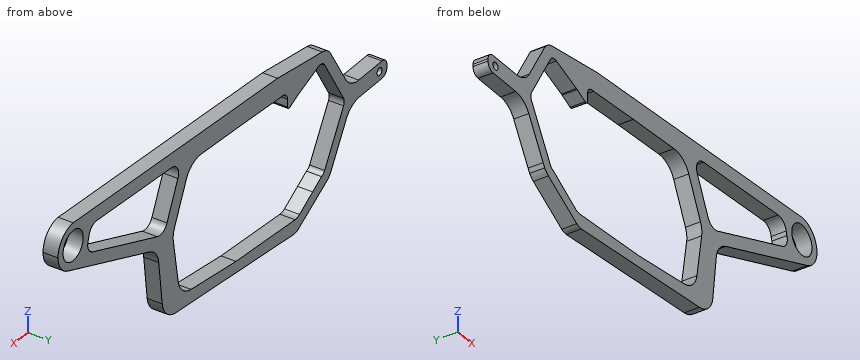
from build123d import *

# Parameters (mm, degrees)
F1_R     = 1
F1_R_2   = 4
F2_DEPTH = 4


# Not quite as in the source:
# - a feature names something its author has since deleted; it is built from what else it names


with BuildPart() as f2:
    # F1 (on Front) → F2 (new body)
    with BuildSketch(Plane.XZ):
        with BuildLine():
            ThreePointArc((53.6725900561, -3.4803708923), (56.4360817028, -1.2749098512), (57.4778270766, 2.1038045583))
            ThreePointArc((57.4778270766, 2.1038045583), (55.7204672392, 6.3464457699), (51.4778255932, 8.1038045583))
            Line((51.4778255932, 8.1038045583), (-29.5767494715, 1.8164854333))
            Line((-29.5767494715, 1.8164854333), (-47.2952228074, -0.9563085456))
            ThreePointArc((-47.2952228074, -0.9563085456), (-48.9181443858, -1.5076422035), (-50.2595064205, -2.5746900675))
            Line((-50.2595064205, -2.5746900675), (-56.5978536574, -13.3921147633))
            ThreePointArc((-56.5978536574, -13.3921147633), (-58.7913353541, -15.5645829823), (-61.7746472195, -16.3588313254))
            Line((-61.7746472195, -16.3588313254), (-70.9623719458, -16.3588313254))
            ThreePointArc((-70.9623719458, -16.3588313254), (-72.3660357626, -16.9341461359), (-72.9621509967, -18.3291034361))
            Line((-72.9621509967, -18.3291034361), (-72.9714351561, -18.9536438246))
            ThreePointArc((-72.9714351561, -18.9536438246), (-72.3963412947, -20.3870355307), (-70.9716561052, -20.9833717139))
            Line((-70.9716561052, -20.9833717139), (-62.0211355409, -20.9833717139))
            ThreePointArc((-62.0211355409, -20.9833717139), (-59.0238889239, -21.7856305971), (-56.8281648814, -23.977867475))
            Line((-56.8281648814, -23.977867475), (-51.1217613336, -33.8375062708))
            Line((-51.1217613336, -33.8375062708), (-50.5134866975, -34.8884954183))
            ThreePointArc((-50.5134866975, -34.8884954183), (-49.834113752, -35.622752626), (-49.0221729234, -36.2070755993))
            Line((-49.0221729234, -36.2070755993), (-37.7895467449, -42.6922353472))
            ThreePointArc((-37.7895467449, -42.6922353472), (-36.9110233024, -43.029081092), (-35.9713694581, -43.0772386209))
            Line((-35.9713694581, -43.0772386209), (10.8377953956, -38.0845412605))
            ThreePointArc((10.8377953956, -38.0845412605), (14.4191592098, -36.3857997297), (16.1597362046, -32.824580657))
            Line((16.1597362046, -32.824580657), (17.5522645357, -21.0756224064))
            ThreePointArc((17.5522645357, -21.0756224064), (18.760112016, -18.1166816586), (21.3157969388, -16.1976453223))
            Line((21.3157969388, -16.1976453223), (53.6725900561, -3.4803708923))
        make_face()
        with Locations((-70.0084173118, -18.6587822488)):
            Circle(F1_R, mode=Mode.SUBTRACT)
        with BuildLine():
            ThreePointArc((-33.5221489054, -5.8863848639), (-32.7820426942, -4.3428905644), (-31.1190403454, -3.9372367165))
            Line((-31.1190403454, -3.9372367165), (-15.3857114758, -2.6969403245))
            ThreePointArc((-15.3857114758, -2.6969403245), (-15.3533597704, -2.6945658839), (-15.320984282, -2.6925413929))
            Line((-15.320984282, -2.6925413929), (0.7603415418, -1.5996367209))
            ThreePointArc((0.7603415418, -1.5996367209), (4.2304854801, -2.4267493449), (6.6177460931, -5.0775984562))
            Line((6.6177460931, -5.0775984562), (11.2725159026, -15.1927708333))
            ThreePointArc((11.2725159026, -15.1927708333), (11.7672314644, -16.8926047847), (11.7443467828, -18.6628181167))
            Line((11.7443467828, -18.6628181167), (9.8637327358, -30.2427322728))
            ThreePointArc((9.8637327358, -30.2427322728), (8.1254532697, -33.5812724587), (4.7405491326, -35.2274468291))
            Line((4.7405491326, -35.2274468291), (-13.1016644536, -37.6254695609))
            Line((-13.1016644536, -37.6254695609), (-36.5010263621, -39.4700978904))
            ThreePointArc((-36.5010263621, -39.4700978904), (-37.4240833549, -39.3995872417), (-38.2816944982, -39.0510057009))
            Line((-38.2816944982, -39.0510057009), (-43.475593846, -35.9307785793))
            Line((-43.475593846, -35.9307785793), (-46.9845830439, -33.8227586638))
            ThreePointArc((-46.9845830439, -33.8227586638), (-47.7169758073, -33.480833261), (-48.2542237632, -32.8769485246))
            Line((-48.2542237632, -32.8769485246), (-55.7535278454, -19.8877718654))
            ThreePointArc((-55.7535278454, -19.8877718654), (-56.0221729234, -18.8865675237), (-55.7535278454, -17.8853631819))
            Line((-55.7535278454, -17.8853631819), (-48.3466238348, -5.0768093424))
            ThreePointArc((-48.3466238348, -5.0768093424), (-47.2942991525, -4.0512417288), (-45.8251853322, -4.0215642922))
            Line((-45.8251853322, -4.0215642922), (-37.9265817129, -6.9582780391))
            Line((-37.9265817129, -6.9582780391), (-37.6259790546, -7.0700425992))
            Line((-37.6259790546, -7.0700425992), (-34.4656276648, -8.5558833842))
            ThreePointArc((-34.4656276648, -8.5558833842), (-33.8292769309, -8.5156852397), (-33.5221489054, -7.9569093245))
            Line((-33.5221489054, -7.9569093245), (-33.5221489054, -5.9059880699))
            ThreePointArc((-33.5221489054, -5.9059880699), (-33.5221729234, -5.8961864669), (-33.5221489054, -5.8863848639))
        make_face(mode=Mode.SUBTRACT)
        with BuildLine():
            ThreePointArc((9.9534750477, -2.9862699605), (10.0919340096, -0.2128411234), (12.4467532901, 1.2588601217))
            Line((12.4467532901, 1.2588601217), (42.0606238873, 3.555977278))
            ThreePointArc((42.0606238873, 3.555977278), (44.1407275048, 2.9281273611), (45.2513978552, 1.0606590347))
            ThreePointArc((45.2513978552, 1.0606590347), (45.3681686541, 0.5136324312), (45.5329001833, -0.0209113441))
            ThreePointArc((45.5329001833, -0.0209113441), (45.4391256015, -2.2717054042), (43.8052859559, -3.8226520781))
            Line((43.8052859559, -3.8226520781), (18.1020868014, -13.9248471934))
            ThreePointArc((18.1020868014, -13.9248471934), (15.884946368, -13.9159482702), (14.2794171364, -12.3868744398))
            Line((14.2794171364, -12.3868744398), (9.9534750477, -2.9862699605))
        make_face(mode=Mode.SUBTRACT)
        with Locations((51.4778270766, 2.1038045583)):
            Circle(F1_R_2, mode=Mode.SUBTRACT)
    extrude(amount=F2_DEPTH)


solid = f2.part
The model under review builds one solid part; all positions refer to its coordinate system, in mm. Give positions to 0.01 mm unless a question says otherwise; leave off trailing zeros. Order: outer loops, then holes, each group sorted by start corner. A loop starts at its lowest first (then second) coordinate and runs counter-clockwise, first axis right, second up. Notation, with made-up numbers: M 49.5,83 L 68.5,83 A23 cw 68.5,121 Z; hole C -14,-4.5 d11. An arc over 180 degrees is marked long. One line per question, with ' | ' between items. Start each with the question number.
1) Consider section C-C, the plane y = -2.7. State how many separate pieces and enclosed holes the cut face has, then the cut area to 3 significant figures.
2) Clearance check with flat-ended pins moving along their axes: P1, Ø12, axis at x = -43, z = -22, coming from the -Y side; P2, Ø1.5, axis at y = -3, z = -10, coming from the -X side; P3, Ø1.5, axis at y = -1, z = -31.5, coming from the +X side. State where each tip first meets the part, or that it passes through.
3) Wall thickness on L1, parallel to Z at x = 1.5, y = -1.2; L2, parallel to Z at x = -37.5, y = -1.1; L3, parallel to X at y = -0.2, z = -27.5: over which ranges is each line inside the solid? List them lowest first. Write a range as from..to.
4) Consider section A-A, the plane z = -22.5. Give the boundary of the cut face in (x, y).
5) Consider section B-B, the plane x = -17.5. Give the boundary of the cut face in (y, z), then the cut area to 3 significant figures.
Found:
1) separate pieces: 1 | enclosed holes: 4 | area: 1,240 mm²
2) P1: passes through | P2: stops at x = -55.05 | P3: stops at x = 16.41
3) L1: z = -39.08..-35.66, -1.6..4.23 | L2: z = -42.84..-39.38, -7.13..0.58 | L3: x = -54.79..-51.36, 10.31..16.79
4) outline: M -58.03,-4 L -54.25,-4 L -54.25,0 L -58.03,0 Z; M 11.12,-4 L 17.38,-4 L 17.38,0 L 11.12,0 Z
5) outline: M -4,-41.11 L 0,-41.11 L 0,-37.97 L -4,-37.97 Z; M -4,-2.86 L 0,-2.86 L 0,2.75 L -4,2.75 Z | area: 35.0 mm²
